Read the model definition and answer for the solid it produces. Units are mm, in the model's axes. Coordinates: 2 decimals unless noted, no trailing zeros. Write each loop counter-clockwise with the first axis right and the second up, starting at its lowest first coordinate (ties: lowest second). Pieces come first, ordered by that corner, then holes. Notation, with made-up numbers: (-12.75, 29.5) -> (7.25, 29.5) arc R20 ccw to (7.25, 38.5) -> close; hole circle Ø11 at (38, 57.25). An arc over 180 degrees is marked (long way). One line per item, written item: value. Start each with the question number.
from build123d import *

# Parameters (mm, degrees)
F1_DEPTH = 20
F2_D     = 5
F3_R     = 2


with BuildPart() as f1:
    # F0 (on Front) → F1 (new body)
    with BuildSketch(Plane.XZ):
        Polygon((26, 0), (0, 0), (0, -10), (26, -22.123999112), align=None)
    extrude(amount=F1_DEPTH)

    # F2 (through all)
    with Locations(Plane(origin=(0, 0, 0), x_dir=(1, 0, 0), z_dir=(0, 1, 0))):
        with Locations((5, 5), (21, 5)):
            Hole(F2_D / 2)

    # F3
    f3_edges = [f1.edges().sort_by_distance(p)[0] for p in [
        (26, -10, -22.123999),
        (0, -10, -10),
        (0, -10, 0),
        (26, -10, 0),
    ]]
    fillet(f3_edges, radius=F3_R)


solid = f1.part
1. Find the intervals of material crossed by probe 1 along X at (y, z) = (-8.75, -7.25); probe 2 along X at (y, z) = (-17, -4.5); probe 3 along Z at (x, y) = (7, -5.5), in increasing order. Write a range as from..to.
2. Given pin 1 (1 mm diameter, centred on x = 4.5, y = -6.5, fed in from -Z); pin 2 (6 mm diameter, centred on x = 11.5, y = -12, fed in from -Z), each flat-ended and moving along its own axis, determine where each tip first touches the part or whether it passes through.
3. A cutting plane is placed at B-B on y = -1.25. Give the vertices of the cut face in (x, z), then the cut area to 3 significant figures.
4. For a pull along Z with two mould halves and no side action, classify faces 1 (the face through (23.5, -10.1, -5.1)), 2 (the face through (2.615, -10.14, -5.751)), 3 (the face through (13, -10, 0)), 4 (the face through (12.001, -9.86, -15.596)) as +Z half, -Z half, draft (parallel to the pull), parting line (faces both ways), or undercut.
5. A cutting plane is placed at D-D on x = 21. Give the vertices of the cut face in (y, z), then the cut area to 3 significant figures.
6. A cutting plane is placed at C-C on x = 7. Give the vertices of the cut face in (y, z).
7. A cutting plane is placed at A-A on z = -6.5. Give the vertices of the cut face in (x, y), then the cut area to 3 significant figures.
Derived:
1. probe 1: x = 0..3.91, 6.09..19.91, 22.09..26
1. probe 2: x = 0..2.55, 7.45..18.55, 23.45..26
1. probe 3: z = -13.26..-6.5, -3.5..0
2. pin 1: stops at z = -12.33
2. pin 2: stops at z = -16.76
3. outline: (0, -8.73) arc R2 ccw to (1.15, -10.54) -> (23.15, -20.8) arc R2 ccw to (26, -18.98) -> (26, -2) arc R2 ccw to (24, 0) -> (2, 0) arc R2 ccw to (0, -2) -> close; hole circle Ø5 at (5, -5); hole circle Ø5 at (21, -5)
3. area: 374 mm2
4. face 1: undercut
4. face 2: undercut
4. face 3: +Z half
4. face 4: -Z half
5. outline: (-20, -19.79) -> (0, -19.79) -> (0, -7.5) -> (-20, -7.5) -> close; (-20, -2.5) -> (0, -2.5) -> (0, 0) -> (-20, 0) -> close
5. area: 296 mm2
6. outline: (-20, -13.26) -> (0, -13.26) -> (0, -6.5) -> (-20, -6.5) -> close; (-20, -3.5) -> (0, -3.5) -> (0, 0) -> (-20, 0) -> close
7. outline: (0, -20) -> (3, -20) -> (3, 0) -> (0, 0) -> close; (7, -20) -> (19, -20) -> (19, 0) -> (7, 0) -> close; (23, -20) -> (26, -20) -> (26, 0) -> (23, 0) -> close
7. area: 360 mm2
